```python
from build123d import *

# Parameters (mm, degrees)
F0_R     = 3.175
F1_DEPTH = 304.8


with BuildPart() as f1:
    # F0 (on Right) → F1 (new body)
    with BuildSketch(Plane.YZ):
        with BuildLine():
            ThreePointArc((-22.8529511317, 51.9202167742), (-13.4157885587, 42.2230655236), (-3.8045140282, 51.7476747914))
            ThreePointArc((-3.8045140282, 51.7476747914), (-12.2986988853, 61.2167320381), (-22.6314001471, 53.7971965969))
            Line((-22.6314001471, 53.7971965969), (-22.8529511317, 51.9202167742))
        make_face()
        with Locations((-13.3295140282, 51.7476747914)):
            Circle(F0_R, mode=Mode.SUBTRACT)
        with BuildLine():
            Line((2.2644576156, 3.968923864), (-3.8045140282, 51.7476747914))
            ThreePointArc((-3.8045140282, 51.7476747914), (-13.4157885587, 42.2230655236), (-22.8529511317, 51.9202167742))
            Line((-22.8529511317, 51.9202167742), (-28.545122604, 3.6961431112))
            ThreePointArc((-28.545122604, 3.6961431112), (-13.2469481423, 15.8743778228), (2.2644576156, 3.968923864))
        make_face()
        with Locations((-9.2709995806, 36.5252)):
            Circle(F0_R, mode=Mode.SUBTRACT)
        with BuildLine():
            Line((-22.8529511317, 51.9202167742), (-22.6314001471, 53.7971965969))
            ThreePointArc((-22.6314001471, 53.7971965969), (-22.78884603, 52.8642154666), (-22.8529511317, 51.9202167742))
        make_face()
        with BuildLine():
            Line((2.7685998529, 0), (2.2644576156, 3.968923864))
            ThreePointArc((2.2644576156, 3.968923864), (-13.2469481423, 15.8743778228), (-28.545122604, 3.6961431112))
            Line((-28.545122604, 3.6961431112), (-28.9814001471, 0))
            Line((-28.9814001471, 0), (-28.6248095933, -3.3458322221))
            ThreePointArc((-28.6248095933, -3.3458322221), (-13.462164486, -15.8710130973), (2.2464969737, -4.0378428646))
            Line((2.2464969737, -4.0378428646), (2.7685998529, 0))
        make_face()
        with Locations((-13.1064001471, 0)):
            Circle(F0_R, mode=Mode.SUBTRACT)
        with BuildLine():
            ThreePointArc((2.7685998529, 0), (2.6420599679, 2.0004072107), (2.2644576156, 3.968923864))
            Line((2.2644576156, 3.968923864), (2.7685998529, 0))
        make_face()
        with BuildLine():
            Line((-28.9814001471, 0), (-28.545122604, 3.6961431112))
            ThreePointArc((-28.545122604, 3.6961431112), (-28.8719534834, 1.8609011253), (-28.9814001471, 0))
        make_face()
        with BuildLine():
            ThreePointArc((2.2464969737, -4.0378428646), (2.637533078, -2.0357287648), (2.7685998529, 0))
            Line((2.7685998529, 0), (2.2464969737, -4.0378428646))
        make_face()
        with BuildLine():
            Line((-28.6248095933, -3.3458322221), (-28.9814001471, 0))
            ThreePointArc((-28.9814001471, 0), (-28.8920007844, -1.6823904185), (-28.6248095933, -3.3458322221))
        make_face()
        with BuildLine():
            Line((-5.3589790656, -62.8571261481), (2.2464969737, -4.0378428646))
            ThreePointArc((2.2464969737, -4.0378428646), (-13.462164486, -15.8710130973), (-28.6248095933, -3.3458322221))
            Line((-28.6248095933, -3.3458322221), (-24.2308362037, -44.5737828668))
            ThreePointArc((-24.2308362037, -44.5737828668), (-26.1909962764, -50.8187140835), (-32.0960141584, -53.6422149647))
            Line((-32.0960141584, -53.6422149647), (-59.3291009865, -54.6148252086))
            ThreePointArc((-59.3291009865, -54.6148252086), (-53.7164409108, -56.9396651329), (-51.3916009865, -62.5523252086))
            ThreePointArc((-51.3916009865, -62.5523252086), (-53.7164409108, -68.1649852842), (-59.3291009865, -70.4898252086))
            Line((-59.3291009865, -70.4898252086), (-15.5585914323, -72.0530576926))
            ThreePointArc((-15.5585914323, -72.0530576926), (-21.3696124649, -55.5810351021), (-5.3541009865, -62.5523252086))
            ThreePointArc((-5.3541009865, -62.5523252086), (-5.3553205843, -62.7047451945), (-5.3589790656, -62.8571261481))
        make_face()
        with BuildLine():
            ThreePointArc((-14.8791009865, -72.0773252086), (-8.2525484872, -69.3944321191), (-5.3589790656, -62.8571261481))
            ThreePointArc((-5.3589790656, -62.8571261481), (-5.3553205843, -62.7047451945), (-5.3541009865, -62.5523252086))
            ThreePointArc((-5.3541009865, -62.5523252086), (-21.3696124649, -55.5810351021), (-15.5585914323, -72.0530576926))
            Line((-15.5585914323, -72.0530576926), (-14.8791009865, -72.0773252086))
        make_face()
        with Locations((-14.8791009865, -62.5523252086)):
            Circle(F0_R, mode=Mode.SUBTRACT)
        with BuildLine():
            ThreePointArc((-15.5585914323, -72.0530576926), (-15.2190628146, -72.0712563962), (-14.8791009865, -72.0773252086))
            Line((-14.8791009865, -72.0773252086), (-15.5585914323, -72.0530576926))
        make_face()
        with BuildLine():
            ThreePointArc((-51.3916009865, -62.5523252086), (-53.7164409108, -56.9396651329), (-59.3291009865, -54.6148252086))
            ThreePointArc((-59.3291009865, -54.6148252086), (-67.2666009865, -62.5523252086), (-59.3291009865, -70.4898252086))
            ThreePointArc((-59.3291009865, -70.4898252086), (-53.7164409108, -68.1649852842), (-51.3916009865, -62.5523252086))
        make_face()
        with Locations((-59.3291009865, -62.5523252086)):
            Circle(F0_R, mode=Mode.SUBTRACT)
    extrude(amount=F1_DEPTH)


solid = f1.part
```
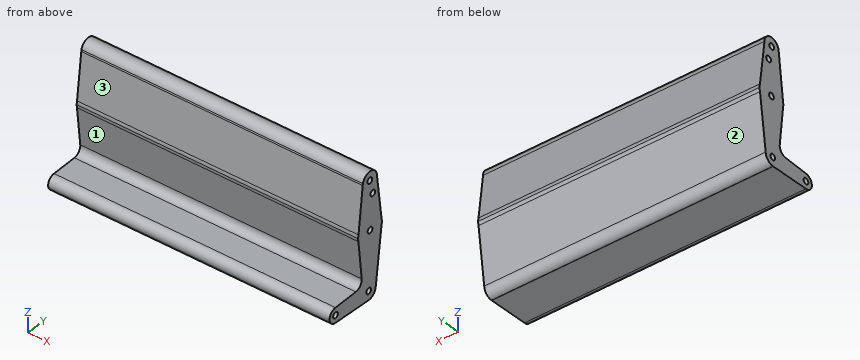
Build history of the part. All positions in model axes, mm. Face numbers are marked on the shaded views. Round coordinates to 2 decimals unless told otherwise and drop trailing zeros. Write each loop counter-clockwise with the first axis right and the second up, starting at its lowest first coordinate (ties: lowest second). Pieces come first, ordered by that corner, then holes. Notation, with made-up numbers: (29.25, -18.75) - (55.25, -18.75) arc R29 cw to (55.25, 18.25) - close; hole circle Ø8 at (-15.5, -40). An arc over 180 degrees is marked (long way). Write each question's results on one line, items separated by ' | '. Start each with the question number.
Item 1: Wall check: L1, parallel to Z at x = 95.5, y = -14; L2, parallel to Y at x = 148, z = 51; L3, parallel to Z at x = 128, y = -41. Give the ranges that are in metal, low to high. Write a range as [from, to].
Item 2: Saw through at A-A (x = 254.5). State how many separate pieces and enclosed holes the cut face has, and give its area (3 significant figures).
Item 3: Saw through at C-C (y = -50). Write the cut outline in (x, z).
Item 4: Mould opens along Z. For the marked faces 1, 2 and 3 say: pulls with the +Z half, pulls with the -Z half, needs draft (parallel to the pull), parting line crosses it, or undercut.
Item 5: Saw through at B-B (z = 7.5). Write the cut outline in (x, y), and give its area (3 significant figures).
Item 6: Drop flat-ended pins along their axis: P1, Ø4, axis at x = 39.5, y = -7.5, coming from the -Z side; P2, Ø7.5, axis at y = -13.11, z = 0, coming from the +X side; P3, Ø5, axis at y = -29.5, z = 19, coming from the -X side; P4, Ø10, axis at x = 152.5, z = -24.5, coming from the +Y side. Give the stop position or say it passes through.
Results are:
1) L1: z = [-72.04, -65.6], [-59.5, -3.05], [3.05, 48.64], [54.85, 61.25] | L2: y = [-22.96, -16.42], [-10.24, -3.71] | L3: z = [-71.14, -53.96]
2) separate pieces: 1 | enclosed holes: 5 | area: 3,710 mm²
3) outline: (0, -70.82) - (304.8, -70.82) - (304.8, -54.28) - (0, -54.28) - close
4) face 1: undercut | face 2: pulls with the -Z half | face 3: pulls with the +Z half
5) outline: (0, -28.1) - (304.8, -28.1) - (304.8, 1.82) - (0, 1.82) - close | area: 9,120 mm²
6) P1: stops at z = -70.41 | P2: stops at x = 304.8 | P3: passes through | P4: stops at y = 0.25
